The listing builds one solid part. Answer for the finished solid, in the listing's coordinates (mm). A direction names the side the tool comes from. Give positions to 0.01 mm unless a question says otherwise; leave off trailing zeros. Write each loop counter-clockwise with the first axis right and the second up, starting at its lowest first coordinate (ties: lowest second). Pieces come first, ordered by that corner, then holes. Notation, with made-up numbers: (-33, 5.25) - (-13, 5.25) arc R23 cw to (-13, 43.25) - close; hole circle Ø8 at (-5.5, 52). An arc over 180 degrees is marked (long way). Use a Markdown table: item, result. Add a question column.
from build123d import *

# Parameters (mm, degrees)
F0_R          = 3.175
F0_R_2        = 1.5875
F1_DEPTH      = 6.35
F1_DEPTH_BACK = 6.35
F0_R_3        = 15.875
F2_DEPTH      = 9.525
F2_DEPTH_BACK = 9.525


with BuildPart() as f1:
    # F0 (on Front) → F1 (new body, two sides)
    with BuildSketch(Plane.XZ) as f1_sk:
        with BuildLine():
            ThreePointArc((7.988833, 20.739556), (18.323515, 12.577734), (22.225, 0))
            ThreePointArc((22.225, 0), (18.472933, -12.357239), (8.483595, -20.542133))
            ThreePointArc((8.483595, -20.542133), (25.28233, -15.682289), (41.413731, -8.929995))
            ThreePointArc((41.413731, -8.929995), (28.577003, -0.195336), (41.044752, 9.05837))
            ThreePointArc((41.044752, 9.05837), (24.886927, 15.946385), (7.988833, 20.739556))
        make_face()
        with BuildLine():
            ThreePointArc((0, 22.225), (4.005284, 21.540726), (7.988833, 20.739556))
            ThreePointArc((7.988833, 20.739556), (4.062881, 21.850483), (0, 22.225))
        make_face()
        with BuildLine():
            ThreePointArc((0, -22.225), (4.324449, -21.800224), (8.483595, -20.542133))
            ThreePointArc((8.483595, -20.542133), (4.253738, -21.443761), (0, -22.225))
        make_face()
        with BuildLine():
            ThreePointArc((-8.030667, 20.723393), (-4.026414, 21.533454), (0, 22.225))
            ThreePointArc((0, 22.225), (-4.084925, 21.846373), (-8.030667, 20.723393))
        make_face()
        with BuildLine():
            ThreePointArc((47.625, 0), (45.806309, 5.598074), (41.044752, 9.05837))
            ThreePointArc((41.044752, 9.05837), (28.577003, -0.195336), (41.413731, -8.929995))
            ThreePointArc((41.413731, -8.929995), (45.919492, -5.438857), (47.625, 0))
        make_face()
        with Locations((38.1, 0)):
            Circle(F0_R, mode=Mode.SUBTRACT)
        with BuildLine():
            ThreePointArc((-8.630772, -20.480732), (-4.402633, -21.784569), (0, -22.225))
            ThreePointArc((0, -22.225), (-4.327986, -21.415212), (-8.630772, -20.480732))
        make_face()
        with BuildLine():
            ThreePointArc((-8.630772, -20.480732), (-22.222643, 0.323655), (-8.030667, 20.723393))
            ThreePointArc((-8.030667, 20.723393), (-24.750865, 15.966198), (-40.743005, 9.150964))
            ThreePointArc((-40.743005, 9.150964), (-32.375011, 7.612498), (-28.575, 0))
            ThreePointArc((-28.575, 0), (-32.294478, -7.551261), (-40.548027, -9.205042))
            ThreePointArc((-40.548027, -9.205042), (-24.903434, -15.731802), (-8.630772, -20.480732))
        make_face()
        with BuildLine():
            ThreePointArc((-28.575, 0), (-32.375011, 7.612498), (-40.743005, 9.150964))
            ThreePointArc((-40.743005, 9.150964), (-47.624463, -0.101169), (-40.548027, -9.205042))
            ThreePointArc((-40.548027, -9.205042), (-32.294478, -7.551261), (-28.575, 0))
        make_face()
        with Locations((-38.1, 0)):
            Circle(F0_R_2, mode=Mode.SUBTRACT)
    extrude(amount=F1_DEPTH)
    extrude(f1_sk.sketch, amount=-F1_DEPTH_BACK)

    # F0 (on Front) → F2 (join, two sides)
    with BuildSketch(Plane.XZ) as f2_sk:
        with BuildLine():
            ThreePointArc((47.625, 0), (45.806309, 5.598074), (41.044752, 9.05837))
            ThreePointArc((41.044752, 9.05837), (28.577003, -0.195336), (41.413731, -8.929995))
            ThreePointArc((41.413731, -8.929995), (45.919492, -5.438857), (47.625, 0))
        make_face()
        with Locations((38.1, 0)):
            Circle(F0_R, mode=Mode.SUBTRACT)
        with BuildLine():
            ThreePointArc((-28.575, 0), (-32.375011, 7.612498), (-40.743005, 9.150964))
            ThreePointArc((-40.743005, 9.150964), (-47.624463, -0.101169), (-40.548027, -9.205042))
            ThreePointArc((-40.548027, -9.205042), (-32.294478, -7.551261), (-28.575, 0))
        make_face()
        with Locations((-38.1, 0)):
            Circle(F0_R_2, mode=Mode.SUBTRACT)
        with BuildLine():
            ThreePointArc((8.483595, -20.542133), (18.472933, -12.357239), (22.225, 0))
            ThreePointArc((22.225, 0), (18.323515, 12.577734), (7.988833, 20.739556))
            ThreePointArc((7.988833, 20.739556), (4.005284, 21.540726), (0, 22.225))
            ThreePointArc((0, 22.225), (-4.026414, 21.533454), (-8.030667, 20.723393))
            ThreePointArc((-8.030667, 20.723393), (-22.222643, 0.323655), (-8.630772, -20.480732))
            ThreePointArc((-8.630772, -20.480732), (-4.327986, -21.415212), (0, -22.225))
            ThreePointArc((0, -22.225), (4.253738, -21.443761), (8.483595, -20.542133))
        make_face()
        Circle(F0_R_3, mode=Mode.SUBTRACT)
    extrude(amount=F2_DEPTH)
    extrude(f2_sk.sketch, amount=-F2_DEPTH_BACK)


solid = f1.part
1. The part is cut by section A-A (y = 7.5). Count the separate pieces of the cut face and the enclosed holes in it, and give its area (3 significant figures).
2. Consider L1, parallel to Z at x = -38.1, y = -8 (1 decimal); L2, parallel to Y at x = 24, z = -11; L3, parallel to X at y = 7.25, z = 2. Determine where each line is inside the solid, lowest interval first. Write a range as [from, to].
3. For a pull along X with two mould halves and no side action, classify faces 1 (the flat face through (25, -6.35, -1)), 2 (the cylindrical face through (-3.97, 7.915, 21.544)), 3 (the flat face through (42, 9.525, 0)) as released by +X, released by -X, zero draft, split by the parting line, or undercut.
4. The part is cut by section B-B (x = -3). Give the vertices of the cut face in (y, z) (3 decimals).
5. Given P1, Ø3, axis at x = 21.5, z = -14, coming from the -Y side; P2, Ø12, axis at x = 17.5, z = -14, coming from the +Y side (3 decimals); P3, Ø6, axis at x = -25.5, z = 1, coming from the +Y side; P4, Ø8, axis at y = -1.5, z = -8, coming from the -X side, each flat-ended and moving along its own axis, determine where each tip first touches the part or whether it passes through.
6. Which of the six approach directions +Z, -Z, +X, -X, +Y, -Y give full straight-line access (tool end or side, diameter ignored) to faces 4 (the cylindrical face through (4.194, -7.915, -21.456)), 5 (the flat face through (4.22, 6.35, -21.63)), 6 (the cylindrical face through (-22.214, -7.915, 0.693))?
Check values:
| question | item | result |
|---|---|---|
| 1 | separate pieces | 3 |
| 1 | enclosed holes | 3 |
| 1 | area | 1,280 mm2 |
| 2 | L1 | z = [-9.5, -1.6], [1.6, 9.5] |
| 2 | L2 | y = [-6.35, 6.35] |
| 2 | L3 | x = [-47.41, -28.79], [-22.13, -15.75], [15.75, 22.13], [28.79, 35.63], [40.57, 47.41] |
| 3 | face 1 | undercut |
| 3 | face 2 | released by -X |
| 3 | face 3 | zero draft |
| 4 | outline | (-9.525, -21.677) - (-6.35, -21.677) - (-6.35, -22.022) - (6.35, -22.022) - (6.35, -21.677) - (9.525, -21.677) - (9.525, -15.589) - (-9.525, -15.589) - close; (-9.525, 15.589) - (9.525, 15.589) - (9.525, 21.721) - (6.35, 21.721) - (6.35, 22.022) - (-6.35, 22.022) - (-6.35, 21.721) - (-9.525, 21.721) - close |
| 5 | P1 | stops at y = -6.35 |
| 5 | P2 | stops at y = 9.525 |
| 5 | P3 | stops at y = 6.35 |
| 5 | P4 | stops at x = -46.74 |
| 6 | face 4 | -Z, +X, -Y |
| 6 | face 5 | -Z, +X, +Y |
| 6 | face 6 | -Y |
